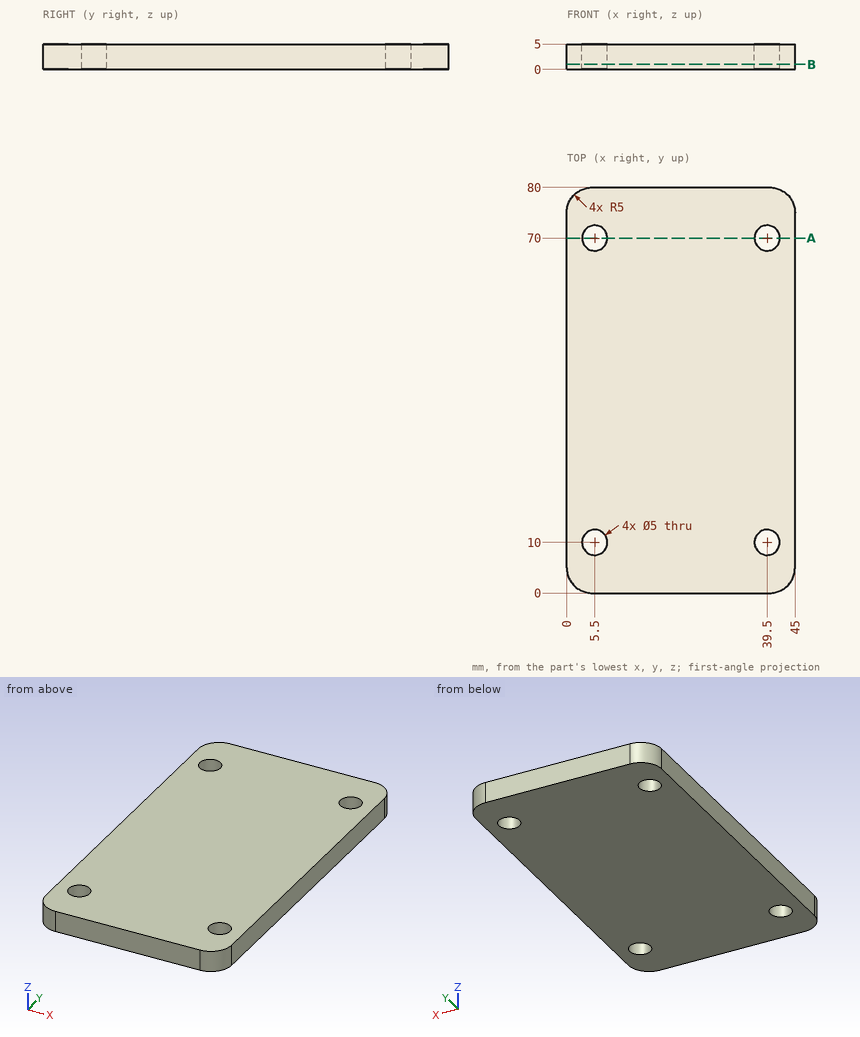
The figure shows three views and two pictorial views of one solid part (mm, origin at its lowest corner). Answer the questions. Coordinates: 2 decimals unless noted, no trailing zeros. Write each loop counter-clockwise with the first axis right and the second up, starting at its lowest first coordinate (ties: lowest second). Pieces come first, ordered by that corner, then holes. Notation, with made-up numbers: (-18, 51.25) -> (34, 51.25) arc R38 ccw to (34, 90.25) -> close; hole circle Ø7 at (85.5, 15.25). An arc over 180 degrees is marked (long way). Return JSON: item names as keys, results as strings.
(1) The part is cut by section B-B on z = 1. Give the vertices of the cut face in (x, y).
Answers below:
{"outline": "(0, 5) arc R5 ccw to (5, 0) -> (40, 0) arc R5 ccw to (45, 5) -> (45, 75) arc R5 ccw to (40, 80) -> (5, 80) arc R5 ccw to (0, 75) -> close; hole circle Ø5 at (5.5, 10); hole circle Ø5 at (5.5, 70); hole circle Ø5 at (39.5, 10); hole circle Ø5 at (39.5, 70)"}
(2) Consider line 1 along Y through (x, z) = (5.5, 1.45); line 2 along X through (y, z) = (70, 1.2); line 3 along Y through (x, z) = (39, 1). Determine where each line is inside the solid, lowest interval first. Write a range as from..to.
Answers below:
{"line 1": "0..7.5, 12.5..67.5, 72.5..80", "line 2": "0..3, 8..37, 42..45", "line 3": "0..7.55, 12.45..67.55, 72.45..80"}
(3) The part is cut by section A-A on y = 70. Give the vertices of the cut face in (x, z), then the cut area to 3 significant figures.
Answers below:
{"outline": "(0, 0) -> (3, 0) -> (3, 5) -> (0, 5) -> close; (8, 0) -> (37, 0) -> (37, 5) -> (8, 5) -> close; (42, 0) -> (45, 0) -> (45, 5) -> (42, 5) -> close", "area": "175 mm^2"}
(4) This flat-tipped pin is pushed along its axis until it touches: P1, Ø4, axis at x = 39.5, y = 70, coming from the -Z side. Where does it stop, or does it pass through?
Answers below:
{"P1": "through"}
